For this review, take the finished solid that the model builds, in its own axes (mm). A direction names the side the tool comes from. Round coordinates to 2 decimals unless told otherwise and drop trailing zeros. Order: outer loops, then holes, each group sorted by start corner. A loop starts at its lowest first (then second) coordinate and runs counter-clockwise, first axis right, second up.
Autodesk Inventor part; units mm, degrees
ref_plane "YZ Plane" through (0, 0, 0) normal (1, 0, 0) x (0, 1, 0)
ref_plane "XZ Plane" through (0, 0, 0) normal (0, 1, 0) x (-1, 0, 0)
ref_plane "XY Plane" through (0, 0, 0) normal (0, 0, 1) x (1, 0, 0)
sketch "Sketch1" plane through (0, 0, 0) normal (0, 1, 0) x (-1, 0, 0)
  circle A0 centre (0, 0) radius 19.05
  circle A1 centre (0, 0) radius 2
  dimension "d0" = 38.1
  dimension "d1" = 4
extrude "Extrusion1" add sketch "Sketch1" along normal blind 2.54
sketch "Sketch2" plane through (0, 2.54, 0) normal (0, 1, 0) x (1, 0, 0)
  circle A0 centre (0, 0) radius 2
  circle A1 centre (0, 0) radius 15.24
  dimension "d4" = 4
  dimension "d5" = 30.48
extrude "Extrusion2" add sketch "Sketch2" along normal blind 7.62
sketch "Sketch3" plane through (0, 10.16, 0) normal (0, 1, 0) x (1, 0, 0)
  circle A0 centre (0, 0) radius 2
  circle A1 centre (0, 0) radius 19.05
  dimension "d8" = 4
  dimension "d9" = 38.1
extrude "Extrusion3" add sketch "Sketch3" along normal blind 2.54
fillet "Fillet1" radius 2.54 1 edges at (-15.24, 10.16, 0)
fillet "Fillet2" radius 2.54 1 edges at (-15.24, 2.54, 0)
properties part number "pulley"
(1) Draft analysis for pull direction Y (two halves, no side actions). For faces 1 (the face through (4, 12.7, 0)), 2 (the face through (15.12, 1.25, 11.59)), 3 (the face through (16, 2.54, 9)), state which applies: pulls with the +Y half, pulls with the -Y half, needs draft (parallel to the pull), parting line crosses it, or undercut.
(2) Clearance check with flat-ended pins moving along their axes: P1, Ø1.5, axis at x = 2.5, y = 10, coming from the -Z side; P2, Ø1.5, axis at x = 12, y = 2, coming from the -Z side; P3, Ø2, axis at x = 5.5, y = 7.5, coming from the -Z side. State where each tip first meets the part, or that it passes through.
(3) Add section C-C on y = 9.5. Give the boundary of the cut face in (x, z).
(4) Wall thickness on L1, parallel to Y at x = 15, z = -9.5; L2, parallel to X at y = 11.9, z = 0; L3, parallel to X at y = 7, z = 0: over which ranges is each line inside the solid? List them lowest first.
(5) Tool access review of faces 4 (the face through (-4, 0, 0)), 5 (the face through (-3.3, 6.33, -14.88)): name each direction out of +Z, -Z, +X, -X, +Y, -Y from which nothing blocks a thin tool from reaching the whole face with its end or side.
(6) Add section B-B on y = 12. Give the boundary of the cut face in (x, z), plus the area to 3 significant figures.
Here are the results:
1. face 1: pulls with the +Y half
1. face 2: needs draft
1. face 3: undercut
2. P1: stops at z = -18.97
2. P2: stops at z = -15.37
2. P3: stops at z = -14.56
3. outline: circle Ø32.14 at (0, 0); hole circle Ø4 at (0, 0)
4. L1: y = 0 to 2.54, 10.16 to 12.7
4. L2: x = -19.05 to -2, 2 to 19.05
4. L3: x = -15.24 to -2, 2 to 15.24
5. face 4: +Z, -Z, +X, -X, -Y
5. face 5: none
6. outline: circle Ø38.1 at (0, 0); hole circle Ø4 at (0, 0)
6. area: 1,130 mm2
